Could you check a few things on this drawing? It's one solid part, dimensions in mm from its lowest x, y, z. A direction names the side the tool comes from. Round coordinates to 2 decimals unless told otherwise and drop trailing zeros. Write each loop counter-clockwise with the first axis right and the second up, starting at its lowest first coordinate (ties: lowest second). Pieces come first, ordered by that corner, then holes. Notation, with made-up numbers: (63.5, -15.75) -> (73.5, -15.75) arc R27 ccw to (73.5, 23.25) -> close; hole circle Ø1 at (-21.75, 80). An arc over 180 degrees is marked (long way). Answer in a Markdown table with one row per item. Add a question column.
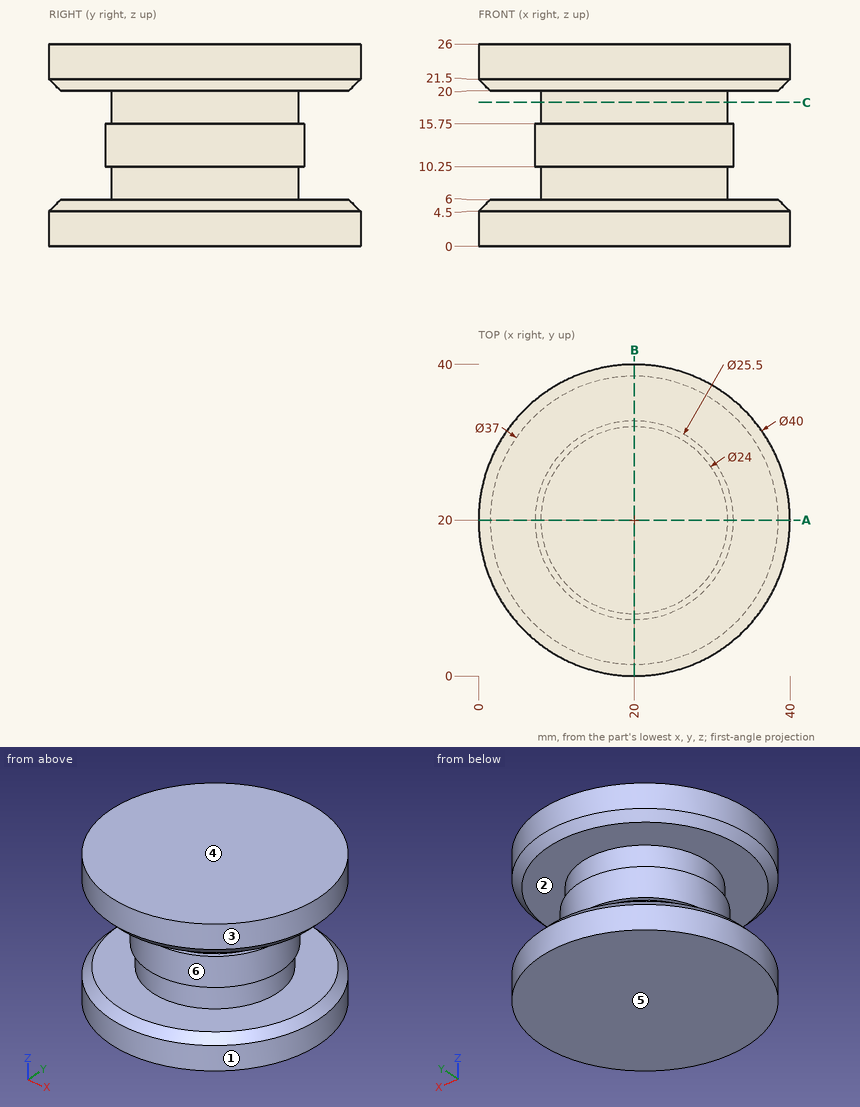
(1) For P1, Ø4, axis at y = 21, z = 10.5, coming from the +X side; P2, Ø10, axis at x = 32.5, z = 8.5, coming from the +Y side; P3, Ø1, axis at x = 21.5, z = 18.5, coming from the -Y side, each with a flat end and sliding along its axis, tell me the tip position at first contact or that it passes through.
(2) On a 3-axis mill with a long thin cutter (end or side, diameter ignored), from which of +Z, -Z, +X, -X, +Y, -Y can I reach the whole of each face in a straight line? I mean the marked faces 1 and 2. Say none if no direction works.
(3) I need wall thicknesses on L1, parallel to Z at x = 36, y = 19; L2, parallel to Z at x = 4.5, y = 8.5; L3, parallel to X at y = 26, z = 9.5. Which ranges of each line are inside material? Lowest first, please.
(4) If we mould it in two halves opening along Z, with no side actions, what happens to the marked faces 3, 4, 5 and 6? For each: pulls with the +Z half, pulls with the -Z half, needs draft (parallel to the pull), parting line crosses it, or undercut.
(5) Suppose I cut it at A-A, the plane y = 20. Please give me the cut outline in (x, z).
(6) Suppose I cut it at C-C, the plane z = 18.5. Please give me the cut outline in (x, y).
Response:
| question | item | result |
|---|---|---|
| 1 | P1 | x = 32.75 |
| 1 | P2 | y = 37.6 |
| 1 | P3 | y = 8.04 |
| 2 | face 1 | +Z, -Z |
| 2 | face 2 | none |
| 3 | L1 | 0 to 6, 20 to 26 |
| 3 | L2 | 0 to 5.2, 20.8 to 26 |
| 3 | L3 | 9.61 to 30.39 |
| 4 | face 3 | needs draft |
| 4 | face 4 | pulls with the +Z half |
| 4 | face 5 | pulls with the -Z half |
| 4 | face 6 | undercut |
| 5 | outline | (0, 0) -> (40, 0) -> (40, 4.5) -> (38.5, 6) -> (32, 6) -> (32, 10.25) -> (32.75, 10.25) -> (32.75, 15.75) -> (32, 15.75) -> (32, 20) -> (38.5, 20) -> (40, 21.5) -> (40, 26) -> (0, 26) -> (0, 21.5) -> (1.5, 20) -> (8, 20) -> (8, 15.75) -> (7.25, 15.75) -> (7.25, 10.25) -> (8, 10.25) -> (8, 6) -> (1.5, 6) -> (0, 4.5) -> close |
| 6 | outline | circle Ø24 at (20, 20) |
